```python
from build123d import *

# Parameters (mm, degrees)
SKETCH1_R             = 6.35
BOSS_EXTRUDE1_DEPTH   = 3.175
FILLET2_R             = 10
FILLET3_R             = 20
M4X0_7_TAPPED_HOLE1_D = 3.3


with BuildPart() as part:
    # Sketch1 → Boss-Extrude1 (new body, symmetric)
    with BuildSketch(Plane.XY):
        Polygon((75.336239509, 30), (-75.336239509, 30), (-95.474630657, 6), (-95.474630657, -6), (-75.336239509, -30), (75.336239509, -30), (95.474630657, -6), (95.474630657, 6), align=None)
        with BuildLine():
            Line((-88.474630657, -1.5875), (-88.474630657, 1.5875))
            ThreePointArc((-88.474630657, 1.5875), (-82.55, 0), (-88.474630657, -1.5875))
        make_face(mode=Mode.SUBTRACT)
        with Locations((-51.435, 0)):
            Circle(SKETCH1_R, mode=Mode.SUBTRACT)
        with Locations((-17.145, 0)):
            Circle(SKETCH1_R, mode=Mode.SUBTRACT)
        with Locations((17.145, 0)):
            Circle(SKETCH1_R, mode=Mode.SUBTRACT)
        with Locations((51.435, 0)):
            Circle(SKETCH1_R, mode=Mode.SUBTRACT)
        with BuildLine():
            ThreePointArc((88.474630657, -1.5875), (82.55, 0), (88.474630657, 1.5875))
            Line((88.474630657, 1.5875), (88.474630657, -1.5875))
        make_face(mode=Mode.SUBTRACT)
    extrude(amount=BOSS_EXTRUDE1_DEPTH, both=True)

    # Fillet2
    fillet2_edges = [part.edges().sort_by_distance(p)[0] for p in [
        (95.474630657, 6, 0),
        (95.474630657, -6, 0),
        (-95.474630657, -6, 0),
        (-95.474630657, 6, 0),
    ]]
    fillet(fillet2_edges, radius=FILLET2_R)

    # Fillet3
    fillet3_edges = [part.edges().sort_by_distance(p)[0] for p in [
        (75.336239509, -30, 0),
        (-75.336239509, -30, 0),
        (-75.336239509, 30, 0),
        (75.336239509, 30, 0),
    ]]
    fillet(fillet3_edges, radius=FILLET3_R)

    # M4x0.7 Tapped Hole1 (through all)
    with Locations(Plane.ZY.offset(95.474630657)):
        with Locations((0, 0)):
            Hole(M4X0_7_TAPPED_HOLE1_D / 2)


solid = part.part
```
The listing builds one solid part. Answer for the finished solid, in the listing's coordinates (mm). Coordinates: 2 decimals unless noted, no trailing zeros. Loops run counter-clockwise (first coordinate to the right, second up) from the corner with the lowest first, then second, coordinate; pieces in that order, holes last. Notation, with made-up numbers: (73, 1) -> (89, 1) arc R6 cw to (89, 9) -> close; hole circle Ø6 at (-32.5, 10). An arc over 180 degrees is marked (long way). Return JSON: item names as keys, results as strings. Group by question number.
(1) Given pin 1 Ø3 at (y, z) = (0, 0) entering from +X, flat-ended and moving along its own axis, determine where the tip first touches the part or whether it passes through.
(2) Find the intervals of material crossed by probe 1 along X at (y, z) = (4.5, 1.25); probe 2 along Y at (x, z) = (1.25, 0); probe 3 along X at (y, z) = (-4, 1), in increasing order. Write a range as from..to.
(3) A cutting plane is placed at C-C on y = -14.5. Write down the section's boundary in (x, z) (3 decimals), and give its area (3 significant figures).
(4) A cutting plane is placed at A-A on x = 18. Write down the section's boundary in (y, z) (3 decimals).
(5) Determine the mould class of faces 1 (the cylindrical face through (-70.112, 1.115, 1.216)), 2 (the flat face through (-1, 0, -3.175)), 3 (the flat face through (-87.32, -15.72, 0.04)) for opening direction Z: released by +Z, released by -Z, zero draft, split by the parting line, or undercut.
(6) A cutting plane is placed at B-B on x = -41. Write down the section's boundary in (y, z) (3 decimals), and give its area (3 significant figures).
(7) A cutting plane is placed at D-D on y = 14. Write down the section's boundary in (x, z) (3 decimals).
The answers:
{
 "1": {"pin 1": "passes through"},
 "2": {"probe 1": "x = -95.24..-55.92, -46.95..-21.63, -12.66..12.66, 21.63..46.95, 55.92..95.24", "probe 2": "y = -30..-1.65, 1.65..30", "probe 3": "x = -95.34..-56.37, -46.5..-22.08, -12.21..12.21, 22.08..46.5, 56.37..95.34"},
 "3": {"outline": "(-88.342, -3.175) -> (88.342, -3.175) -> (88.342, 3.175) -> (-88.342, 3.175) -> close", "area": "1,120 mm^2"},
 "4": {"outline": "(-30, -3.175) -> (-6.292, -3.175) -> (-6.292, 3.175) -> (-30, 3.175) -> close; (6.292, -3.175) -> (30, -3.175) -> (30, 3.175) -> (6.292, 3.175) -> close"},
 "5": {"face 1": "undercut", "face 2": "released by -Z", "face 3": "zero draft"},
 "6": {"outline": "(-30, -3.175) -> (30, -3.175) -> (30, 3.175) -> (-30, 3.175) -> close; hole circle Ø3.3 at (0, 0)", "area": "372 mm^2"},
 "7": {"outline": "(-88.762, -3.175) -> (88.762, -3.175) -> (88.762, 3.175) -> (-88.762, 3.175) -> close"}
}
